Study the drawing (mm; zero at the part's minimum x, y, z) and answer. A direction names the side the tool comes from. Round coordinates to 2 decimals unless told otherwise and drop trailing zeros. Loops run counter-clockwise (first coordinate to the right, second up) from the corner with the lowest first, then second, coordinate; pieces in that order, holes last. Notation, with made-up numbers: (40.25, 41) -> (93.25, 41) arc R15 ccw to (93.25, 66) -> close; hole circle Ø5 at (43.25, 62). An arc over 180 degrees is marked (long way). Answer in a Markdown table with one row per item. Add a question column.
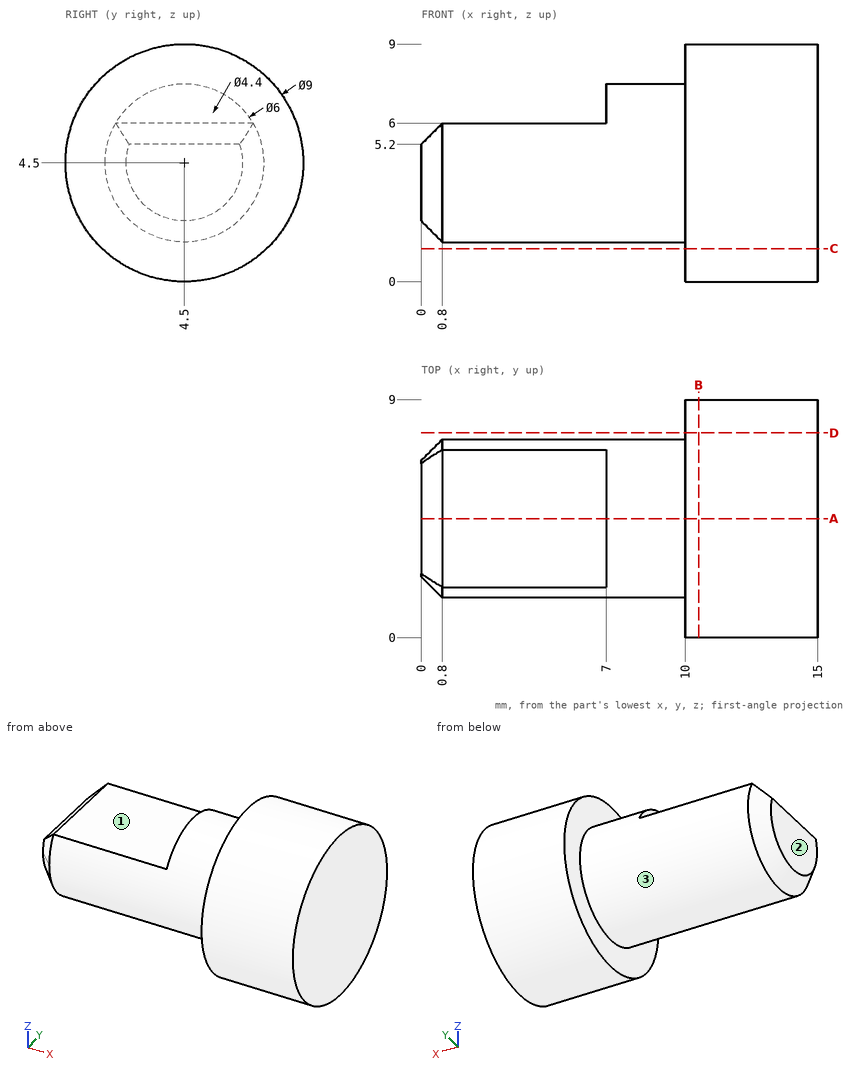
Item 1: Section B-B, the plane x = 10.5 is taken. Write down the section's boundary in (y, z).
Item 2: Section A-A, the plane y = 4.5 is taken. Write down the section's boundary in (x, z), and give its area (3 significant figures).
Item 3: Section C-C, the plane z = 1.25 is taken. Write down the section's boundary in (x, y), and give its area (3 significant figures).
Item 4: For the marked faces 1, 2 and 3, determine the directions among +Z, -Z, +X, -X, +Y, -Y from which every point of the face is accessible in a straight line to the end or side of a thin tool.
Item 5: Flat-ended cylindrical pins translate along their axes: P1, Ø5, axis at x = 2.5, z = 5.5, coming from the +Y side; P2, Ø2, axis at x = 4, y = 5.5, coming from the -Z side; P3, Ø2, axis at x = 8.5, y = 2.5, coming from the -Z side. Find the tip coordinate at first contact, or state that the pin passes through.
Item 6: Consider L1, parallel to Z at x = 6.5, y = 6; L2, parallel to X at y = 4, z = 1.5; L3, parallel to X at y = 3, z = 6.75. Determine where each line is inside the solid, lowest interval first. Write a range as from..to.
Here are the results:
| question | item | result |
|---|---|---|
| 1 | outline | circle Ø9 at (4.5, 4.5) |
| 2 | outline | (0, 2.3) -> (0.8, 1.5) -> (10, 1.5) -> (10, 0) -> (15, 0) -> (15, 9) -> (10, 9) -> (10, 7.5) -> (7, 7.5) -> (7, 6) -> (0.8, 6) -> (0, 5.2) -> close |
| 2 | area | 93.9 mm² |
| 3 | outline | (10, 1.39) -> (15, 1.39) -> (15, 7.61) -> (10, 7.61) -> close |
| 3 | area | 31.1 mm² |
| 4 | face 1 | +Z, -X, +Y, -Y |
| 4 | face 2 | +Z, -Z, -X, +Y, -Y |
| 4 | face 3 | -X |
| 5 | P1 | stops at y = 7.5 |
| 5 | P2 | stops at z = 1.5 |
| 5 | P3 | stops at z = 1.67 |
| 6 | L1 | z = 1.9..6 |
| 6 | L2 | x = 10..15 |
| 6 | L3 | x = 7..15 |
